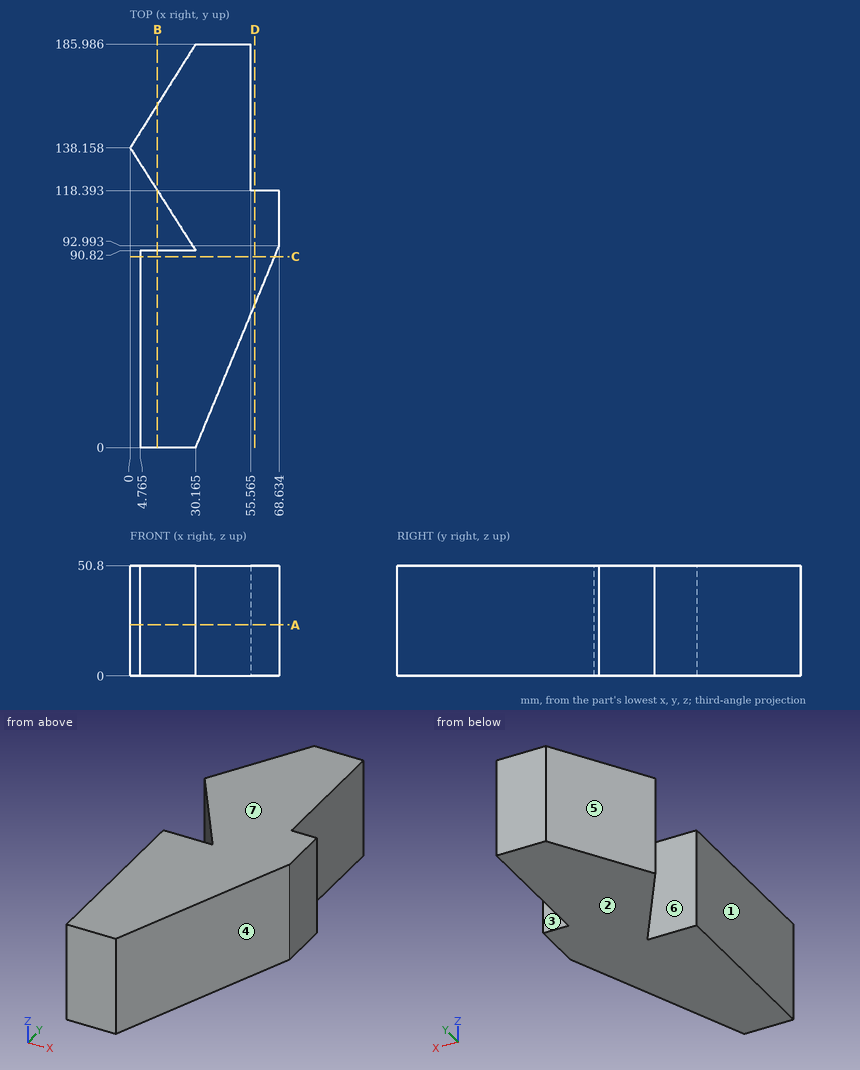
Geometry: see drawing. Coordinates: mm, zero at the bounding-box minimum. A direction names the side the tool comes from. Round coordinates to 2 decimals unless told otherwise and drop trailing zeros. Order: outer loops, then holes, each group sorted by start corner. A loop starts at its lowest first (then second) coordinate and runs counter-clockwise, first axis right, second up. Notation, with made-up numbers: (-36, 59.5) - (-16, 59.5) arc R23 cw to (-16, 73.5) - close; hole circle Ø7 at (59.5, -11.75). An arc over 180 degrees is marked (long way). Use a Markdown table: item, result. Add a question column.
1. Section query B-B (x = 12.5). Return the cut outline in (y, z), then the cut area to 3 significant figures.
2. Section query A-A (z = 23.5). Return the cut outline in (x, y) (1 decimal).
3. Section query D-D (x = 57.5). Return the cut outline in (y, z), then the cut area to 3 significant figures.
4. Section query C-C (y = 88). Return the cut outline in (x, z) (1 decimal), then the cut area to 3 significant figures.
5. Mould query, pull axis Y, two halves, no side actions, for the marked faces 4, 5, 6 and 7. Classes: +Y half, -Y half, draft (parallel to the pull), parting line (faces both ways), or undercut.
6. Set-up query: the marked faces 1, 2 and 3. Return all of +Z, -Z, +X, -X, +Y, -Y with unobstructed straight access to the full face (end or side cutting, diameter ignored); none if empty.
7. Line query: probe 1 along Y at (x, z) = (5, 15) (1 decimal); probe 2 along Y at (x, z) = (23.5, 23.5) (1 decimal); probe 3 along X at (y, z) = (9.5, 15) (1 decimal). Output: solid intervals per line, ascending.
8. First-contact query: pin 1 (10 mm diameter, centred on y = 84.5, z = 5.5, fed in from -X) (1 decimal); pin 2 (20.5 mm diameter, centred on x = 15, z = 21.5, fed in from +Y) (1 decimal); pin 3 (2 mm diameter, centred on y = 58.5, z = 41, fed in from +X). Flat tips, straight axial feed; report the tip coordinate or a pass-through.
Derived:
| question | item | result |
|---|---|---|
| 1 | outline | (0, 0) - (90.82, 0) - (90.82, 50.8) - (0, 50.8) - close; (118.54, 0) - (157.98, 0) - (157.98, 50.8) - (118.54, 50.8) - close |
| 1 | area | 6,620 mm2 |
| 2 | outline | (0, 138.2) - (30.2, 90.8) - (4.8, 90.8) - (4.8, 0) - (30.2, 0) - (68.6, 93) - (68.6, 118.4) - (55.6, 118.4) - (55.6, 186) - (30.2, 186) - close |
| 3 | outline | (66.08, 0) - (118.39, 0) - (118.39, 50.8) - (66.08, 50.8) - close |
| 3 | area | 2,660 mm2 |
| 4 | outline | (4.8, 0) - (66.6, 0) - (66.6, 50.8) - (4.8, 50.8) - close |
| 4 | area | 3,140 mm2 |
| 5 | face 4 | -Y half |
| 5 | face 5 | +Y half |
| 5 | face 6 | undercut |
| 5 | face 7 | draft |
| 6 | face 1 | +Z, -Z, -X, -Y |
| 6 | face 2 | -Z, +X, -X, +Y, -Y |
| 6 | face 3 | +Z, -Z, +X, +Y |
| 7 | probe 1 | 0 to 90.8, 130.3 to 146.1 |
| 7 | probe 2 | 0 to 90.8, 101.3 to 175.4 |
| 7 | probe 3 | 4.8 to 34.1 |
| 8 | pin 1 | x = 4.8 |
| 8 | pin 2 | y = 178.2 |
| 8 | pin 3 | x = 54.78 |
